Job drawing, mm, ordinate dimensions from the low corner. One solid piece. Round coordinates to 2 decimals unless told otherwise and drop trailing zeros. Write each loop counter-clockwise with the first axis right and the second up, starting at its lowest first coordinate (ties: lowest second). Pieces come first, ordered by that corner, then holes. Notation, with made-up numbers: M 83.25,-2 L 141.25,-2 A27 ccw 141.25,17 Z; hole C 48.5,-36.5 d1. An arc over 180 degrees is marked long. One line per item, written item: value. Start each with the question number.
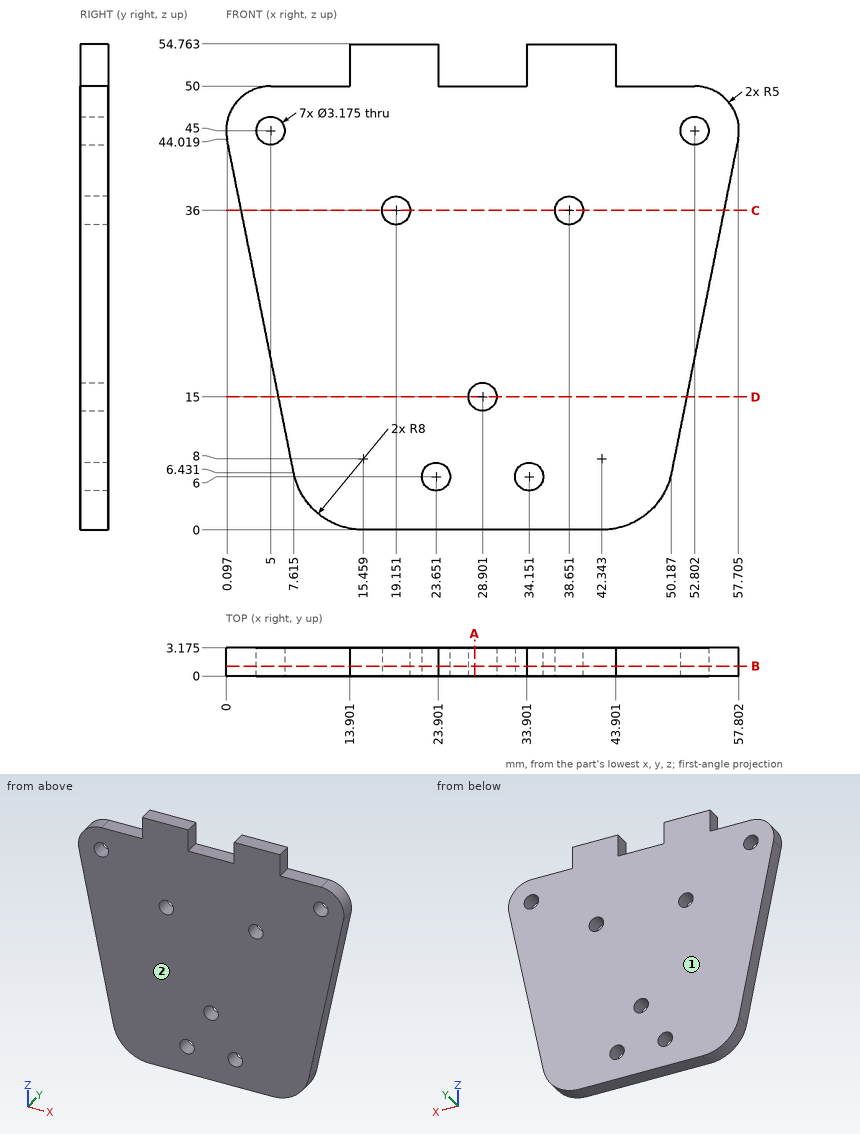
Item 1: Drop flat-ended pins along their axis: pin 1 (1.6 mm diameter, centred on x = 11, y = 2, fed in from +Z); pin 2 (1.6 mm diameter, centred on y = 2, z = 51.5, fed in from -X); pin 3 (1.6 mm diameter, centred on y = 2, z = 53, fed in from +X). Give the stop position or say it passes through.
Item 2: Two-plate mould, pull along Y, no slides. Class the marked faces 1 and 2: pulls with the +Y half, pulls with the -Y half, needs draft (parallel to the pull), parting line crosses it, or undercut.
Item 3: Cut at C-C, the plane z = 36. Write the cut outline in (x, y) (1 decimal).
Item 4: Drill centre lines: line 1 (X direction, y = 1.9, z = 45.5) (1 decimal); line 2 (X direction, y = 1.45, z = 36); line 3 (Z direction, x = 43.5, y = 2.4) (1 decimal). Where is each one in solid material? Low to high.
Item 5: Cut at B-B, the plane y = 1.1. Count the separate pieces of the cut face and the enclosed holes in it, plus the area to 3 significant figures.
Item 6: Cut at D-D, the plane z = 15. Write the cut outline in (x, y) (1 decimal).
Item 7: Cut at A-A, the plane x = 28. Write the cut outline in (y, z) (1 decimal).
Computed values:
1. pin 1: stops at z = 50
1. pin 2: stops at x = 13.9
1. pin 3: stops at x = 43.9
2. face 1: pulls with the +Y half
2. face 2: pulls with the -Y half
3. outline: M 1.7,0 L 17.6,0 L 17.6,3.2 L 1.7,3.2 Z; M 20.7,0 L 37.1,0 L 37.1,3.2 L 20.7,3.2 Z; M 40.2,0 L 56.1,0 L 56.1,3.2 L 40.2,3.2 Z
4. line 1: x = 0 to 3.5, 6.5 to 51.3, 54.3 to 57.8
4. line 2: x = 1.7 to 17.56, 20.74 to 37.06, 40.24 to 56.1
4. line 3: z = 0.1 to 54.8
5. separate pieces: 1
5. enclosed holes: 7
5. area: 2,510 mm2
6. outline: M 5.9,0 L 27.3,0 L 27.3,3.2 L 5.9,3.2 Z; M 30.5,0 L 51.9,0 L 51.9,3.2 L 30.5,3.2 Z
7. outline: M 0,0 L 3.2,0 L 3.2,13.7 L 0,13.7 Z; M 0,16.3 L 3.2,16.3 L 3.2,50 L 0,50 Z
